For this review, use the dimensioned drawing (mm, ordinates from the lowest corner) and the shaded views. A direction names the side the tool comes from. Coordinates: 2 decimals unless noted, no trailing zeros. Loops run counter-clockwise (first coordinate to the right, second up) from the corner with the lowest first, then second, coordinate; pieces in that order, holes last. Notation, with made-up numbers: M 78.25,45 L 129.25,45 A18 cw 129.25,56 Z; hole C 68.25,83.5 d3. An arc over 180 degrees is marked long. One line per item, written item: value.
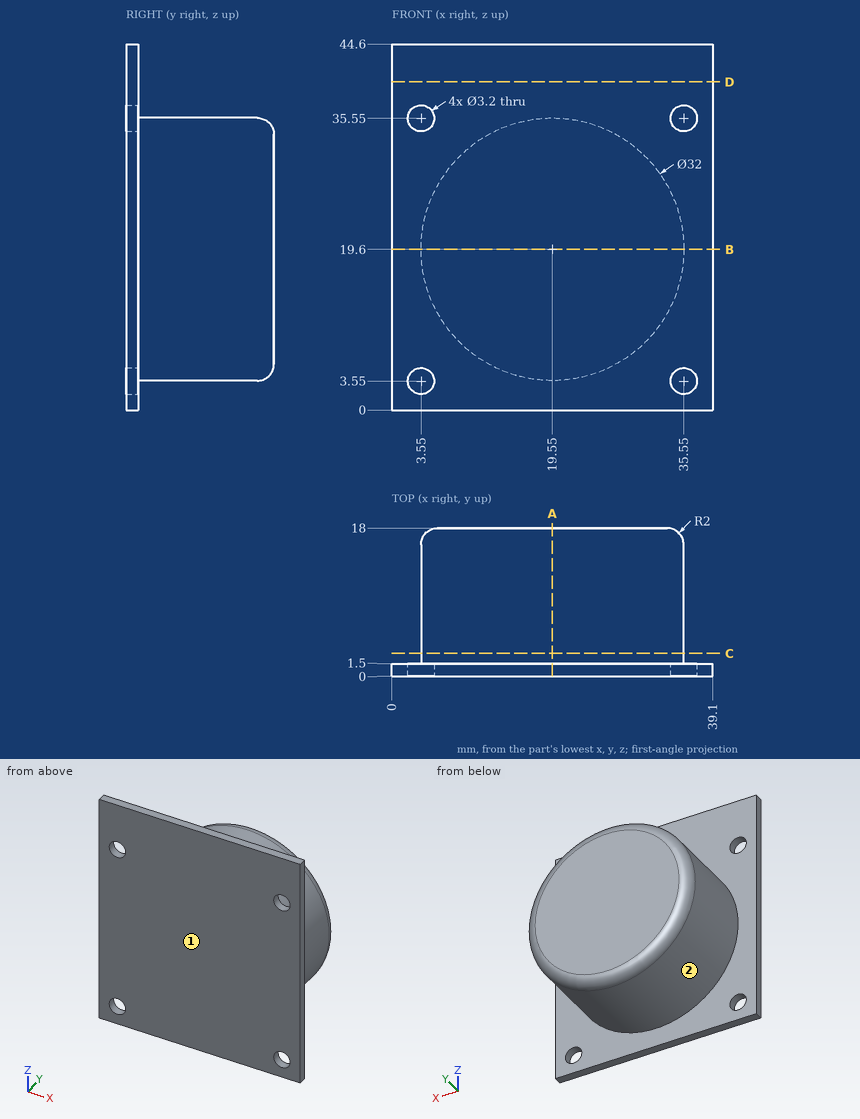
(1) Add section B-B on z = 19.6. State the section outline as (x, y) points, then the cut area to 3 significant figures.
Checks:
outline: M 0,0 L 39.1,0 L 39.1,1.5 L 35.55,1.5 L 35.55,16 A2 ccw 33.55,18 L 5.55,18 A2 ccw 3.55,16 L 3.55,1.5 L 0,1.5 Z
area: 585 mm^2
(2) To check wall thickness, follow L1, parallel to Z at x = 35.55, y = 1.05; L2, parallel to X at y = 0.95, z = 35.55; L3, parallel to Z at x = 20, y = 11.75. State the ranges of each line that lie inside material, in increasing order. Write a range as [from, to].
Checks:
L1: [0, 1.95], [5.15, 33.95], [37.15, 44.6]
L2: [0, 1.95], [5.15, 33.95], [37.15, 39.1]
L3: [3.61, 35.59]
(3) Add section A-A on x = 19.55. State the section outline as (y, z) points.
Checks:
outline: M 0,0 L 1.5,0 L 1.5,3.6 L 16,3.6 A2 ccw 18,5.6 L 18,33.6 A2 ccw 16,35.6 L 1.5,35.6 L 1.5,44.6 L 0,44.6 Z
(4) Add section C-C on y = 2.75. State the section outline as (x, z) points.
Checks:
outline: C 19.55,19.6 d32
(5) Insertion check: pin 1 Ø8 at (x, y) = (12.5, 10.5) entering from -Z; pin 2 Ø4 at (x, z) = (35.55, 3.55) entering from +Y; pin 3 Ø3 at (y, z) = (14, 8.5) entering from +X; pin 4 Ø2.5 at (x, z) = (3.55, 3.55) entering from -Y. Each pin has a flat end and moves straight along its axis. Give the tip position at first contact, or say it passes through.
Checks:
pin 1: z = 3.89
pin 2: y = 1.5
pin 3: x = 32.35
pin 4: through
(6) Add section D-D on z = 40. State the section outline as (x, y) points.
Checks:
outline: M 0,0 L 39.1,0 L 39.1,1.5 L 0,1.5 Z
(7) Tool access review of the marked faces 1 and 2: name each direction out of +Z, -Z, +X, -X, +Y, -Y from which nothing blocks a thin tool from reaching the whole face with its end or side.
Checks:
face 1: +Z, -Z, +X, -X, -Y
face 2: +Y
